Geometry: final body of the model. Coordinates: model frame, mm. Face numbers are marked on the shaded views. Give positions to 0.01 mm unless a question says otherwise; leave off trailing zeros. Order: outer loops, then holes, each group sorted by start corner. A loop starts at its lowest first (then second) coordinate and runs counter-clockwise, first axis right, second up. Notation, with made-up numbers: (-23.5, 86.5) -> (6.5, 86.5) arc R19 cw to (6.5, 93.5) -> close; hole circle Ø1 at (11, -11.75). An arc over 180 degrees is marked (long way). Write item = value, one per line.
```python
from build123d import *

# Parameters (mm, degrees)
SKETCH1_R           = 1.016
BOSS_EXTRUDE1_DEPTH = 47.371
SKETCH2_R           = 2.4892
BOSS_EXTRUDE2_DEPTH = 4.699
SKETCH3_W           = 6.35
SKETCH3_H           = 6.35
BOSS_EXTRUDE3_DEPTH = 1.651
SKETCH4_R           = 2.4892
BOSS_EXTRUDE4_DEPTH = 10.16
BOSS_EXTRUDE5_START = 4.699
SKETCH5_R           = 2.4892
BOSS_EXTRUDE5_DEPTH = 4.699
SKETCH6_W           = 6.35
SKETCH6_H           = 6.35
BOSS_EXTRUDE6_DEPTH = 1.651
BOSS_EXTRUDE7_START = 10.16
SKETCH7_R           = 2.4892
BOSS_EXTRUDE7_DEPTH = 10.16


with BuildPart() as part:
    # Sketch1 → Boss-Extrude1 (new body)
    with BuildSketch(Plane.XY):
        Circle(SKETCH1_R)
    extrude(amount=BOSS_EXTRUDE1_DEPTH)

    # Sketch2 → Boss-Extrude2 (add)
    with BuildSketch(Plane(origin=(0, 0, 0), x_dir=(-1, 0, 0), z_dir=(0, 0, -1))):
        Circle(SKETCH2_R)
    extrude(amount=BOSS_EXTRUDE2_DEPTH)

    # Sketch3 → Boss-Extrude3 (add)
    with BuildSketch(Plane(origin=(0, 0, -4.699), x_dir=(-1, 0, 0), z_dir=(0, 0, -1))):
        Rectangle(SKETCH3_W, SKETCH3_H)
    extrude(amount=BOSS_EXTRUDE3_DEPTH)

    # Sketch4 → Boss-Extrude4 (add)
    with BuildSketch(Plane(origin=(0, 0, -6.35), x_dir=(-1, 0, 0), z_dir=(0, 0, -1))):
        Circle(SKETCH4_R)
    extrude(amount=BOSS_EXTRUDE4_DEPTH)

    # Sketch5 → Boss-Extrude5 (add)
    with BuildSketch(Plane.XY.offset(47.371).offset(BOSS_EXTRUDE5_START)):
        with Locations(Location((0, 0, 0), (0, 0, 180))):
            Circle(SKETCH5_R)
    extrude(amount=-BOSS_EXTRUDE5_DEPTH)

    # Sketch6 → Boss-Extrude6 (add)
    with BuildSketch(Plane.XY.offset(52.07)):
        Rectangle(SKETCH6_W, SKETCH6_H)
    extrude(amount=BOSS_EXTRUDE6_DEPTH)

    # Sketch7 → Boss-Extrude7 (add)
    with BuildSketch(Plane.XY.offset(53.721).offset(BOSS_EXTRUDE7_START)):
        with Locations(Location((0, 0, 0), (0, 0, 180))):
            Circle(SKETCH7_R)
    extrude(amount=-BOSS_EXTRUDE7_DEPTH)


solid = part.part
```
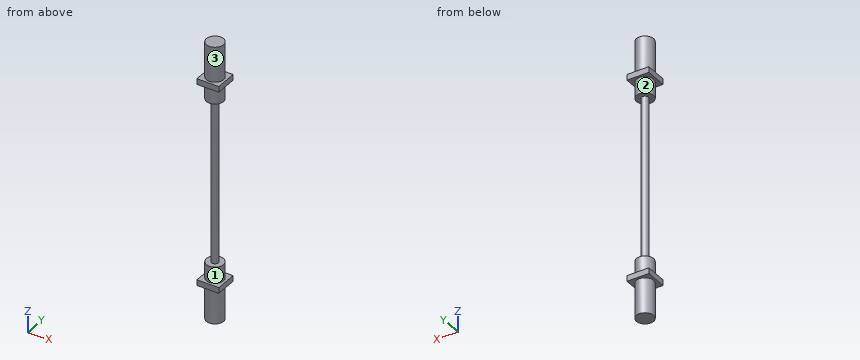
1) Section query D-D (z = -7). Output: boundary loops of the cut face in (x, y).
Check sheet entries:
outline = circle Ø4.98 at (0, 0)
2) Section query C-C (z = 11). Output: boundary loops of the cut face in (x, y), plus the area to 3 significant figures.
Check sheet entries:
outline = circle Ø2.03 at (0, 0)
area = 3.24 mm²
3) Mould query, pull axis Z, two halves, no side actions, for the marked faces 1, 2 and 3. Classes: +Z half, -Z half, draft (parallel to the pull), parting line (faces both ways), or undercut.
Check sheet entries:
face_1 = undercut
face_2 = undercut
face_3 = draft
4) First-contact query: P1, Ø3, axis at x = 2, z = -7.5, coming from the +Y side (3 decimals); P2, Ø1, axis at y = 2, z = 26, coming from the -X side. Flat tips, straight axial feed; report the tip coordinate or a pass-through.
Check sheet entries:
P1 = 3.175
P2 = through
5) Line query: line 1 (Z direction, x = 1.25, y = -2.25); line 2 (Y direction, x = 0, z = 9); line 3 (Z direction, x = -0.25, y = 1.5). Output: solid intervals per line, ascending. Write a range as from..to.
Check sheet entries:
line_1 = -6.35..-4.7, 52.07..53.72
line_2 = -1.02..1.02
line_3 = -16.51..0, 47.37..63.88
6) Section query A-A (x = 0). Output: boundary loops of the cut face in (y, z) (3 decimals).
Check sheet entries:
outline = (-3.175, -6.35) -> (-2.489, -6.35) -> (-2.489, -16.51) -> (2.489, -16.51) -> (2.489, -6.35) -> (3.175, -6.35) -> (3.175, -4.699) -> (2.489, -4.699) -> (2.489, 0) -> (1.016, 0) -> (1.016, 47.371) -> (2.489, 47.371) -> (2.489, 52.07) -> (3.175, 52.07) -> (3.175, 53.721) -> (2.489, 53.721) -> (2.489, 63.881) -> (-2.489, 63.881) -> (-2.489, 53.721) -> (-3.175, 53.721) -> (-3.175, 52.07) -> (-2.489, 52.07) -> (-2.489, 47.371) -> (-1.016, 47.371) -> (-1.016, 0) -> (-2.489, 0) -> (-2.489, -4.699) -> (-3.175, -4.699) -> close
